```python
from build123d import *

# Parameters (mm, degrees)
F0_R          = 4.445
F0_R_2        = 2.8448
F1_DEPTH      = 12.7
F2_DEPTH      = 304.8
F4_DEPTH      = 25.4
F4_DEPTH_BACK = 25.4


with BuildPart() as f1:
    # F0 (on Right) → F1 (new body)
    with BuildSketch(Plane.YZ):
        Circle(F0_R)
        Circle(F0_R_2, mode=Mode.SUBTRACT)
    extrude(amount=-F1_DEPTH)

    # F0 (on Right) → F2 (join)
    with BuildSketch(Plane.YZ):
        Circle(F0_R)
        Circle(F0_R_2, mode=Mode.SUBTRACT)
    extrude(amount=-F2_DEPTH)

    # F3 (on Front) → F4 (cut, two sides)
    with BuildSketch(Plane.XZ) as f4_sk:
        Polygon((-253.9987727039, -0.0183600185), (-259.0788954335, -0.0148181376), (-259.0788954335, -1.7928185265), (-254.0000123471, -1.7963595863), align=None)
        Polygon((-259.0788954335, 1.7631822513), (-259.0788954335, -0.0148181376), (-253.9987727039, -0.0183600185), (-253.9975330607, 1.7596395494), align=None)
        Polygon((-269.2391408927, 1.7702659267), (-269.2391408927, -0.0077343758), (-264.1590181631, -0.0112762567), (-264.1590181631, 1.766724089), align=None)
        Polygon((-264.1590181631, -0.0112762567), (-269.2391408927, -0.0077343758), (-269.2391408927, -1.7857346783), (-264.1590181631, -1.7892766024), align=None)
        Polygon((-279.3993863519, 1.7773496021), (-279.3993863519, -0.000650614), (-274.3192636223, -0.0041924949), (-274.3192636223, 1.7738077644), align=None)
        Polygon((-274.3192636223, -0.0041924949), (-279.3993863519, -0.000650614), (-279.3993863519, -1.7786508301), (-274.3192636223, -1.7821927542), align=None)
        Polygon((-284.4795090815, 0.0028912669), (-289.5596318112, 0.0064331478), (-289.5608714541, -1.7715661175), (-284.4807487246, -1.7751080416), align=None)
        Polygon((-289.5583921682, 1.7844324132), (-289.5596318112, 0.0064331478), (-284.4795090815, 0.0028912669), (-284.4782694385, 1.7808905755), align=None)
        Polygon((-294.6397545408, 0.0099750287), (-299.7198772704, 0.0135169096), (-299.7198772704, -1.7644831336), (-294.6409941837, -1.7680241934), align=None)
        Polygon((-299.7198772704, 1.7915169528), (-299.7198772704, 0.0135169096), (-294.6397545408, 0.0099750287), (-294.6385148978, 1.7879742509), align=None)
    extrude(amount=-F4_DEPTH, mode=Mode.SUBTRACT)
    extrude(f4_sk.sketch, amount=F4_DEPTH_BACK, mode=Mode.SUBTRACT)


solid = f1.part
```
Source: CAD feature listing. Evaluate the final solid. Frame: model axes, mm. Coordinates: 2 decimals unless noted, no trailing zeros. Loops run counter-clockwise (first coordinate to the right, second up) from the corner with the lowest first, then second, coordinate; pieces in that order, holes last. Notation, with made-up numbers: (-30, 51) - (29, 51) arc R15 ccw to (29, 63) - close; hole circle Ø8 at (4, -12). An arc over 180 degrees is marked (long way). Answer as CSV lines item,"result".
1. Section B-B (x = -50). Return loops of the section in (y, z) (3 decimals), then the cut area to 3 significant figures.
Established:
outline,"circle Ø8.89 at (0, 0); hole circle Ø5.69 at (0, 0)"
area,"36.6 mm2"
2. Ray query, line 1 (X direction, y = 3.25, z = 0.5); line 2 (Z direction, x = -194, y = 0) (3 decimals); line 3 (Y direction, x = -50, z = 0.5). Return the intervals inside material, ascending.
Established:
line 1,"x = -304.8 to -299.72, -294.64 to -289.56, -284.48 to -279.4, -274.32 to -269.24, -264.16 to -259.08, -254 to 0"
line 2,"z = -4.445 to -2.845, 2.845 to 4.445"
line 3,"y = -4.42 to -2.8, 2.8 to 4.42"
3. Mould query, pull axis Y, two halves, no side actions, for faces 1 (the cylindrical face through (-150.27, -0.37, 2.82)), 2 (the cylindrical face through (-150.27, -4.44, 0.2)), 3 (the flat face through (-304.8, 0, -3)). Classes: released by +Y, released by -Y, zero draft, split by the parting line, or undercut.
Established:
face 1,"undercut"
face 2,"split by the parting line"
face 3,"zero draft"
4. Contact query for flat-ended pins moving along their axis: pin 1 (1.5 mm diameter, centred on x = -75, y = 3.5, fed in from +Z); pin 2 (4 mm diameter, centred on x = -201, y = 3, fed in from -Z); pin 3 (1 mm diameter, centred on y = -0.5, z = 0.5, fed in from -X) (3 decimals). Output: stop coordinate, or through.
Established:
pin 1,"stops at z = 3.49"
pin 2,"stops at z = -4.33"
pin 3,"passes through"
5. Section A-A (y = 0). Return loops of the section in (x, z) (3 decimals), then the cut area to 3 significant figures.
Established:
outline,"(-304.8, -4.445) - (0, -4.445) - (0, -2.845) - (-304.8, -2.845) - close; (-304.8, 2.845) - (0, 2.845) - (0, 4.445) - (-304.8, 4.445) - close"
area,"975 mm2"
